from build123d import *

# Parameters (mm, degrees)
SKETCH1_W                  = 26.3
SKETCH1_H                  = 26.3
SKETCH1_W_2                = 20.3
SKETCH1_H_2                = 20.3
TUBE_EXTRUDE_DEPTH         = 60
HEX_EXTRUDE_DEPTH          = 26.3
SKETCH3_W                  = 23.3
SKETCH3_H                  = 26.968911086
TUBE_CENTER_CUT_DEPTH      = 1
TUBE_CENTER_CUT_DEPTH_BACK = 27.3
CUT_EXTRUDE1_START         = -3
CUT_EXTRUDE1_DEPTH         = 3
SKETCH5_W                  = 1
SKETCH5_H                  = 10.515544457
CUT_EXTRUDE2_DEPTH         = 27.3
FILLET1_R                  = 3
FILLET2_R                  = 1
SKETCH6_W                  = 23.3
SKETCH6_H                  = 60
CUT_EXTRUDE3_DEPTH         = 27.3


with BuildPart() as part:
    # Sketch1 → Tube Extrude (new body)
    with BuildSketch(Plane(origin=(0, 0, 0), x_dir=(1, 0, 0), z_dir=(0, 1, 0))):
        with Locations((10.15, 10.15)):
            Rectangle(SKETCH1_W, SKETCH1_H)
        with Locations((10.15, 10.15)):
            Rectangle(SKETCH1_W_2, SKETCH1_H_2, mode=Mode.SUBTRACT)
    extrude(amount=TUBE_EXTRUDE_DEPTH)

    # Sketch2 → Hex Extrude (add)
    with BuildSketch(Plane.XY.offset(3)):
        Polygon((23.3, 15.649519053), (23.3, 0), (36.852881057, -7.824759526), (49.655762114, -0.433012702), (62.45864317, -7.824759526), (75.261524227, -0.433012702), (88.064405284, -7.824759526), (100.867286341, -0.433012702), (113.670167397, -7.824759526), (127.223048454, 0), (127.223048454, 15.649519053), (127.223048454, 44.350480947), (127.223048454, 60), (113.670167397, 67.824759526), (100.867286341, 60.433012702), (88.064405284, 67.824759526), (75.261524227, 60.433012702), (62.45864317, 67.824759526), (49.655762114, 60.433012702), (36.852881057, 67.824759526), (23.3, 60), (23.3, 44.350480947), align=None)
        Polygon((49.655762114, 16.082531755), (37.602881057, 23.041265877), (37.602881057, 36.958734123), (49.655762114, 43.917468245), (61.70864317, 36.958734123), (61.70864317, 23.041265877), align=None, mode=Mode.SUBTRACT)
        Polygon((36.102881057, 23.041265877), (24.8, 16.515544457), (24.8, 43.484455543), (36.102881057, 36.958734123), align=None, mode=Mode.SUBTRACT)
        Polygon((24.8, 0.866025404), (36.852881057, -6.092708719), (48.905762114, 0.866025404), (48.905762114, 14.783493649), (36.852881057, 21.742227772), (24.8, 14.783493649), align=None, mode=Mode.SUBTRACT)
        Polygon((50.405762114, 0.866025404), (62.45864317, -6.092708719), (74.511524227, 0.866025404), (74.511524227, 14.783493649), (62.45864317, 21.742227772), (50.405762114, 14.783493649), align=None, mode=Mode.SUBTRACT)
        Polygon((76.011524227, 0.866025404), (88.064405284, -6.092708719), (100.117286341, 0.866025404), (100.117286341, 14.783493649), (88.064405284, 21.742227772), (76.011524227, 14.783493649), align=None, mode=Mode.SUBTRACT)
        Polygon((125.723048454, 16.515544457), (114.420167397, 23.041265877), (114.420167397, 36.958734123), (125.723048454, 43.484455543), align=None, mode=Mode.SUBTRACT)
        Polygon((101.617286341, 0.866025404), (113.670167397, -6.092708719), (125.723048454, 0.866025404), (125.723048454, 14.783493649), (113.670167397, 21.742227772), (101.617286341, 14.783493649), align=None, mode=Mode.SUBTRACT)
        Polygon((24.8, 45.216506351), (36.852881057, 38.257772228), (48.905762114, 45.216506351), (48.905762114, 59.133974596), (36.852881057, 66.092708719), (24.8, 59.133974596), align=None, mode=Mode.SUBTRACT)
        Polygon((50.405762114, 45.216506351), (62.45864317, 38.257772228), (74.511524227, 45.216506351), (74.511524227, 59.133974596), (62.45864317, 66.092708719), (50.405762114, 59.133974596), align=None, mode=Mode.SUBTRACT)
        Polygon((76.011524227, 45.216506351), (88.064405284, 38.257772228), (100.117286341, 45.216506351), (100.117286341, 59.133974596), (88.064405284, 66.092708719), (76.011524227, 59.133974596), align=None, mode=Mode.SUBTRACT)
        Polygon((101.617286341, 45.216506351), (113.670167397, 38.257772228), (125.723048454, 45.216506351), (125.723048454, 59.133974596), (113.670167397, 66.092708719), (101.617286341, 59.133974596), align=None, mode=Mode.SUBTRACT)
        Polygon((75.261524227, 16.082531755), (87.314405284, 23.041265877), (87.314405284, 36.958734123), (75.261524227, 43.917468245), (63.20864317, 36.958734123), (63.20864317, 23.041265877), align=None, mode=Mode.SUBTRACT)
        Polygon((100.867286341, 16.082531755), (112.920167397, 23.041265877), (112.920167397, 36.958734123), (100.867286341, 43.917468245), (88.814405284, 36.958734123), (88.814405284, 23.041265877), align=None, mode=Mode.SUBTRACT)
    extrude(amount=-HEX_EXTRUDE_DEPTH)

    # Sketch3 → Tube Center Cut (cut, two sides)
    with BuildSketch(Plane.XY.offset(3)) as tube_center_cut_sk:
        with Locations((8.65, 30)):
            Rectangle(SKETCH3_W, SKETCH3_H)
    extrude(amount=TUBE_CENTER_CUT_DEPTH, mode=Mode.SUBTRACT)
    extrude(tube_center_cut_sk.sketch, amount=-TUBE_CENTER_CUT_DEPTH_BACK, mode=Mode.SUBTRACT)

    # Sketch4 → Cut-Extrude1 (cut)
    with BuildSketch(Plane.ZY.offset(3).offset(CUT_EXTRUDE1_START)):
        Polygon((-10.15, 60), (-10.35, 60), (-10.35, 0), (-10.15, 0), (-9.95, 0), (-9.95, 60), align=None)
    extrude(amount=CUT_EXTRUDE1_DEPTH, mode=Mode.SUBTRACT)

    # Sketch5 → Cut-Extrude2 (cut, through all)
    with BuildSketch(Plane.XY.offset(3)):
        with Locations((-2.5, 51.742227771)):
            Rectangle(SKETCH5_W, SKETCH5_H)
        with Locations((-2.5, 8.257772229)):
            Rectangle(SKETCH5_W, SKETCH5_H)
    extrude(amount=-CUT_EXTRUDE2_DEPTH, mode=Mode.SUBTRACT)

    # Fillet1
    fillet1_edges = [part.edges().sort_by_distance(p)[0] for p in [
        (-2, 51.742227772, -23.3),
        (-2, 51.742227772, 3),
        (-2, 8.257772228, -23.3),
        (-2, 8.257772228, 3),
        (24.8, 52.175240474, -23.3),
        (24.8, 52.175240474, 3),
        (24.8, 7.824759526, -23.3),
        (24.8, 7.824759526, 3),
        (24.8, 30, 3),
        (24.8, 30, -23.3),
    ]]
    fillet(fillet1_edges, radius=FILLET1_R)

    # Fillet2
    fillet2_edges = [part.edges().sort_by_distance(p)[0] for p in [
        (0, 0, -15.325),
        (10.15, 0, 0),
        (20.3, 0, -10.15),
        (10.15, 0, -20.3),
        (0, 60, -15.325),
        (10.15, 60, 0),
        (20.3, 60, -10.15),
        (10.15, 60, -20.3),
        (10.15, 43.484455543, -20.3),
        (10.15, 16.515544457, -20.3),
        (-3, 15.015544457, -23.3),
        (-3, 15.015544457, 3),
        (20.3, 30, 3),
        (10.15, 16.515544457, 0),
        (0, 16.515544457, -4.975),
        (0, 43.484455543, -15.325),
        (10.15, 43.484455543, 0),
        (20.3, 30, -23.3),
        (0, 43.484455543, -4.975),
        (0, 16.515544457, -15.325),
        (0, 60, -4.975),
        (0, 0, -4.975),
        (-3, 1.5, -23.3),
        (-3, 44.984455543, -23.3),
        (-3, 1.5, 3),
        (-3, 44.984455543, 3),
        (-3, 58.5, -23.3),
        (-3, 58.5, 3),
    ]]
    fillet(fillet2_edges, radius=FILLET2_R)

    # Sketch6 → Cut-Extrude3 (cut, through all)
    with BuildSketch(Plane.XY.offset(3)):
        with Locations((8.65, 30)):
            Rectangle(SKETCH6_W, SKETCH6_H)
    extrude(amount=-CUT_EXTRUDE3_DEPTH, mode=Mode.SUBTRACT)


solid = part.part
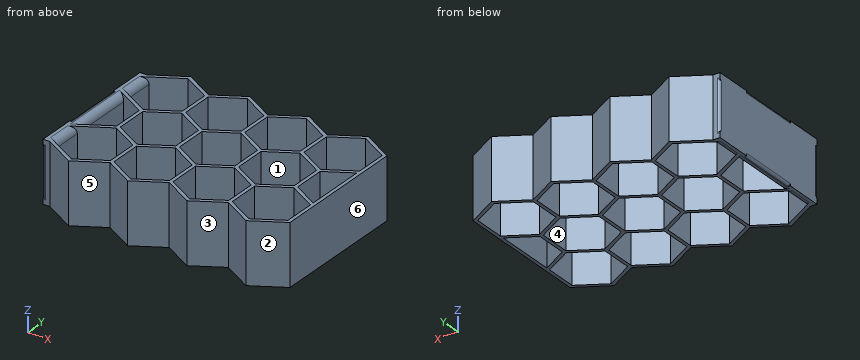
Input: part model. Units: mm. Frame: model coordinates. Face numbers are marked on the shaded views. A direction names the side the tool comes from. Coordinates: 2 decimals unless noted, no trailing zeros. Loops run counter-clockwise (first coordinate to the right, second up) from the corner with the lowest first, then second, coordinate; pieces in that order, holes last. Notation, with made-up numbers: (-0.5, 64) -> (5.5, 64) arc R15 ccw to (5.5, 76) -> close; hole circle Ø10 at (25.5, -0.5). An arc over 180 degrees is marked (long way). One line per item, written item: value.
(1) Cut plane C-C (z = -1.25). Give the number of separate pieces and of enclosed holes in the cut face, then the cut area to 3 significant figures.
Answer below:
separate pieces: 1
enclosed holes: 13
area: 1,260 mm2
(2) Set-up query: the marked faces 1, 2 and 3. Return all of +Z, -Z, +X, -X, +Y, -Y with unobstructed straight access to the full face (end or side cutting, diameter ignored); none if empty.
Answer below:
face 1: +Z, -Z
face 2: +Z, -Z, +X, -Y
face 3: +Z, -Z, -Y
(3) Pin query (flat end, axial travel): pin 1 Ø5 at (x, z) = (47, -18.5) entering from -Y; pin 2 Ø4 at (x, y) = (98, 49) entering from +Z; pin 3 Ø12 at (x, z) = (58, -12.5) entering from +Y; pin 4 Ø0.9 at (x, z) = (21.5, -5) entering from -Y. Return the tip coordinate at first contact, or that it passes through.
Answer below:
pin 1: stops at y = -3.41
pin 2: passes through
pin 3: stops at y = 67.82
pin 4: stops at y = 0
(4) Cut plane A-A (y = 29). Output: boundary loops of the cut face in (x, z), then the cut area to 3 significant figures.
Answer below:
outline: (20.3, -22.3) arc R1 ccw to (21.3, -23.3) -> (21.8, -23.3) arc R3 ccw to (24.8, -20.3) -> (24.8, 0) arc R3 ccw to (21.8, 3) -> (21.3, 3) arc R1 ccw to (20.3, 2) -> close; (36.1, -23.3) -> (37.6, -23.3) -> (37.6, 3) -> (36.1, 3) -> close; (61.71, -23.3) -> (63.21, -23.3) -> (63.21, 3) -> (61.71, 3) -> close; (87.31, -23.3) -> (88.81, -23.3) -> (88.81, 3) -> (87.31, 3) -> close; (112.92, -23.3) -> (114.42, -23.3) -> (114.42, 3) -> (112.92, 3) -> close; (125.72, -23.3) -> (127.22, -23.3) -> (127.22, 3) -> (125.72, 3) -> close
area: 311 mm2
(5) Draft query along Y for the marked faces 4, 5 and 6. Return one class per face: pulls with the +Y half, pulls with the -Y half, needs draft (parallel to the pull), parting line crosses it, or undercut.
Answer below:
face 4: undercut
face 5: pulls with the -Y half
face 6: needs draft
(6) Ray query, line 1 along X through (y, z) = (10, -13); line 2 along X through (y, z) = (24, -5.5); line 3 along Y through (x, z) = (71.5, -13.5). Return the intervals inside material, ascending.
Answer below:
line 1: x = 20.3 to 24.8, 48.91 to 50.41, 74.51 to 76.01, 100.12 to 101.62, 125.72 to 127.22
line 2: x = 20.3 to 24.8, 36.1 to 37.6, 61.71 to 63.21, 87.31 to 88.81, 112.92 to 114.42, 125.72 to 127.22
line 3: y = -2.6 to -0.87, 16.52 to 18.25, 41.75 to 43.48, 60.87 to 62.6
(7) Cut plane B-B (x = 56). Output: boundary loops of the cut face in (y, z).
Answer below:
outline: (-4.1, -23.3) -> (-2.36, -23.3) -> (-2.36, 3) -> (-4.1, 3) -> close; (18.01, -23.3) -> (19.75, -23.3) -> (19.75, 3) -> (18.01, 3) -> close; (40.25, -23.3) -> (41.99, -23.3) -> (41.99, 3) -> (40.25, 3) -> close; (62.36, -23.3) -> (64.1, -23.3) -> (64.1, 3) -> (62.36, 3) -> close
